Design review of the part built by this model. Coordinates are the model's own, in mm. Give positions to 0.01 mm unless a question says otherwise; leave off trailing zeros. Loops run counter-clockwise (first coordinate to the right, second up) from the corner with the lowest first, then second, coordinate; pieces in that order, holes last.
from build123d import *

# Parameters (mm, degrees)
S01_OUTER_RACE_RETAINING_LIP_R          = 22
S01_OUTER_RACE_RETAINING_LIP_R_2        = 12
F_01_OUTER_RACE_RETAINING_LIP_DEPTH     = 2
F_02_START                              = -1
S02_THREE_ACCESSIBLE_SCREW_HOLES_R      = 1.7
F_02_THREE_ACCESSIBLE_SCREW_HOLES_DEPTH = 4


with BuildPart() as part:
    # S01 - Outer race retaining lip → 01 - Outer race retaining lip (new body)
    with BuildSketch(Plane.XY):
        Circle(S01_OUTER_RACE_RETAINING_LIP_R)
        Circle(S01_OUTER_RACE_RETAINING_LIP_R_2, mode=Mode.SUBTRACT)
    extrude(amount=F_01_OUTER_RACE_RETAINING_LIP_DEPTH)

    # S02 - Three accessible screw holes → 02 - Three accessible screw holes (cut)
    with BuildSketch(Plane.XY.offset(F_02_START)):
        with Locations((0, 18.25)):
            Circle(S02_THREE_ACCESSIBLE_SCREW_HOLES_R)
        with Locations((-15.804963619, -9.125)):
            Circle(S02_THREE_ACCESSIBLE_SCREW_HOLES_R)
        with Locations((15.804963619, -9.125)):
            Circle(S02_THREE_ACCESSIBLE_SCREW_HOLES_R)
    extrude(amount=F_02_THREE_ACCESSIBLE_SCREW_HOLES_DEPTH, mode=Mode.SUBTRACT)


solid = part.part
Q1. Take a section at B-B (y = 0). Give the boundary of the cut face in (x, z).
Results:
outline: (-22, 0) - (-12, 0) - (-12, 2) - (-22, 2) - close; (12, 0) - (22, 0) - (22, 2) - (12, 2) - close
Q2. Draft analysis for pull direction Y (two halves, no side actions). For faces 1 (the face through (9, -9, 0)), 2 (the face through (-0.221, 19.936, 0.986)), 3 (the face through (-15.021, -10.633, 0.986)), 4 (the face through (-4.769, -21.477, 0.986)), state which applies: pulls with the +Y half, pulls with the -Y half, needs draft (parallel to the pull), parting line crosses it, or undercut.
Results:
face 1: needs draft
face 2: undercut
face 3: undercut
face 4: parting line crosses it
Q3. Take a section at A-A (x = 0). Give the boundary of the cut face in (y, z), plus the area to 3 significant figures.
Results:
outline: (-22, 0) - (-12, 0) - (-12, 2) - (-22, 2) - close; (12, 0) - (16.55, 0) - (16.55, 2) - (12, 2) - close; (19.95, 0) - (22, 0) - (22, 2) - (19.95, 2) - close
area: 33.2 mm2
Q4. Take a section at C-C (x = 11). Give the boundary of the cut face in (y, z), plus the area to 3 significant figures.
Results:
outline: (-19.05, 0) - (-4.8, 0) - (-4.8, 2) - (-19.05, 2) - close; (4.8, 0) - (19.05, 0) - (19.05, 2) - (4.8, 2) - close
area: 57.0 mm2
Q5. Wall thickness on line 1 (X direction, y = -10, z = 0.95); line 2 (Y direction, x = 1.5, z = 0.85); line 3 (X direction, y = -11, z = 1.45): over which ranges is each line inside the solid? List them lowest first.
Results:
line 1: x = -19.6 to -17.26, -14.35 to -6.63, 6.63 to 14.35, 17.26 to 19.6
line 2: y = -21.95 to -11.91, 11.91 to 17.45, 19.05 to 21.95
line 3: x = -19.05 to -4.8, 4.8 to 19.05
Q6. Insertion check: pin 1 (3 mm diameter, centred on x = -13, y = -5.5, fed in from -Z); pin 2 (1 mm diameter, centred on y = -14.5, z = 0.5, fed in from -X). Each pin has a flat end and moves straight along its axis. Give the tip position at first contact, or say it passes through.
Results:
pin 1: stops at z = 0
pin 2: stops at x = -16.97
Q7. Take a section at D-D (z = 0.8). Give the boundary of the cut face in (x, y) (3 decimals), plus the area to 3 significant figures.
Results:
outline: circle Ø44 at (0, 0); hole circle Ø3.4 at (-15.805, -9.125); hole circle Ø24 at (0, 0); hole circle Ø3.4 at (0, 18.25); hole circle Ø3.4 at (15.805, -9.125)
area: 1,040 mm2
